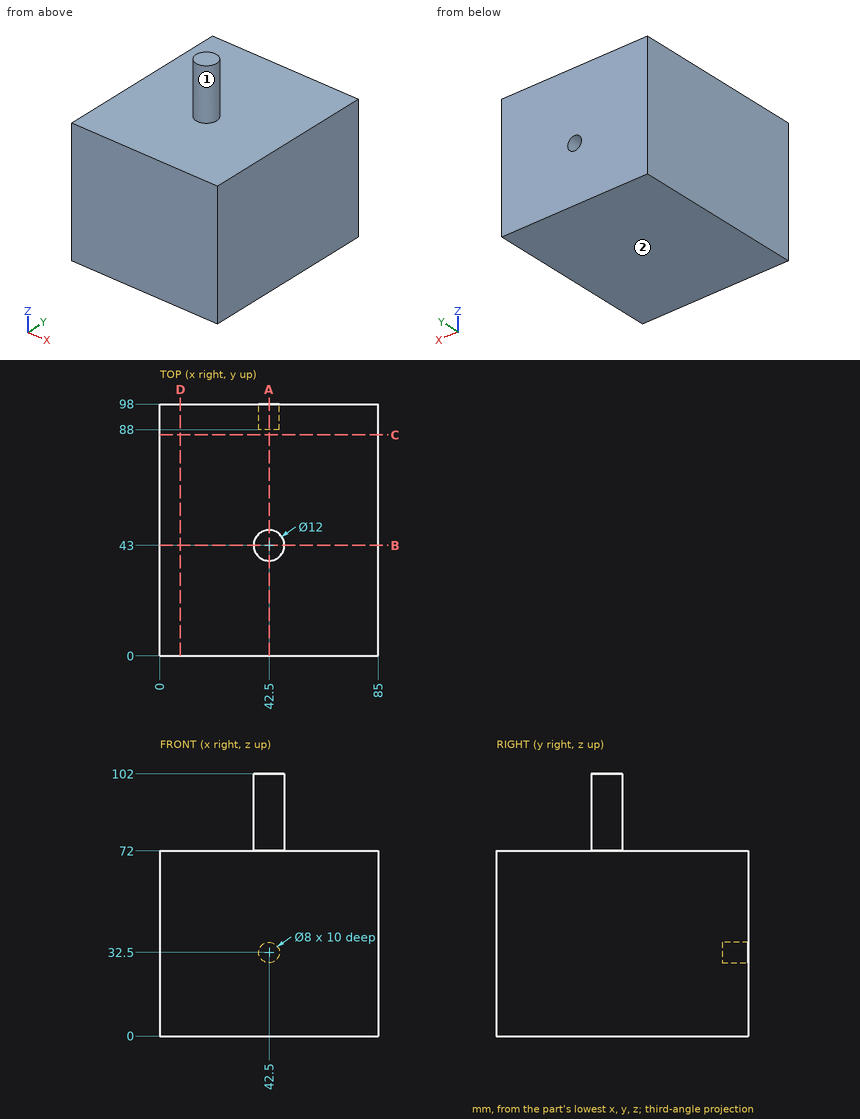
Verification items for this drawing (mm, ordinates from the low corner). A direction names the side the tool comes from. Coordinates: 2 decimals unless noted, no trailing zeros. Order: outer loops, then holes, each group sorted by start corner. A loop starts at its lowest first (then second) coordinate and runs counter-clockwise, first axis right, second up. Notation, with made-up numbers: M -12.75,-33 L 5.25,-33 A14 ccw 5.25,-6 Z; hole C 11,-5.5 d5. An arc over 180 degrees is marked long. Use CSV: the item, a comma, the result in double quotes.
Item 1: Cross-section at D-D on x = 8. Record the cut outline in (y, z), then the cut area to 3 significant figures.
Returned:
outline,"M 0,0 L 98,0 L 98,72 L 0,72 Z"
area,"7,060 mm2"
Item 2: Cross-section at A-A on x = 42.5. Record the cut outline in (y, z), then the cut area to 3 significant figures.
Returned:
outline,"M 0,0 L 98,0 L 98,28.5 L 88,28.5 L 88,36.5 L 98,36.5 L 98,72 L 49,72 L 49,102 L 37,102 L 37,72 L 0,72 Z"
area,"7,340 mm2"
Item 3: Thickness scan on line 1 along Z through (x, y) = (42, 95); line 2 along X through (y, z) = (93, 32.5); line 3 along Z through (x, y) = (8.5, 26). Record the ranges inside material, lowest first.
Returned:
line 1,"z = 0 to 28.53, 36.47 to 72"
line 2,"x = 0 to 38.5, 46.5 to 85"
line 3,"z = 0 to 72"
Item 4: Cross-section at C-C on y = 86. Record the cut outline in (x, z), then the cut area to 3 significant figures.
Returned:
outline,"M 0,0 L 85,0 L 85,72 L 0,72 Z"
area,"6,120 mm2"
Item 5: Cross-section at B-B on y = 43. Record the cut outline in (x, z).
Returned:
outline,"M 0,0 L 85,0 L 85,72 L 48.5,72 L 48.5,102 L 36.5,102 L 36.5,72 L 0,72 Z"
Item 6: Tool access check on the marked faces 1 and 2. Record the directions out of +Z, -Z, +X, -X, +Y, -Y that give a thin tool (end or side, any length) a straight path to the whole face; none if there is none.
Returned:
face 1,"+Z"
face 2,"-Z, +X, -X, +Y, -Y"
Item 7: Gauge pin test, flat ends, axial feed: pin 1 Ø4 at (x, y) = (44.5, 47) entering from -Z; pin 2 Ø6.5 at (x, z) = (42.5, 32.5) entering from +Y. Record the tip position at first contact, or that the pin passes through.
Returned:
pin 1,"stops at z = 0"
pin 2,"stops at y = 88"
